Work out the finished part from the listing and answer in its coordinate system (mm). Round coordinates to 2 decimals unless told otherwise and drop trailing zeros. Write each loop counter-clockwise with the first axis right and the second up, starting at its lowest first coordinate (ties: lowest second). Pieces come first, ordered by that corner, then holes.
1. Straight lines are drawn through the part: probe 1 along Y at (x, z) = (99.9, 0); probe 2 along X at (y, z) = (11.75, 0); probe 3 along Z at (x, y) = (28.5, 15). For each, find the intervals that lie inside material, in ascending order.
2. Find section B-B (z = 70). Write down the section's boundary in (x, y).
3. Determine the mould class of faces 1 (the face through (-22.025, 12.522, 99.184)), 2 (the face through (-21.199, 12.878, 95.465)), 3 (the face through (-53, 0, -83)) for opening direction X: pulls with the +X half, pulls with the -X half, needs draft (parallel to the pull), parting line crosses it, or undercut.
4. Find section A-A (x = -28.5). Write down the section's boundary in (y, z).
5. Flat-ended cylindrical pins translate along their axes: pin 1 Ø8 at (x, y) = (-51, 14.5) entering from -Z; pin 2 Ø4 at (y, z) = (19, -23) entering from +X; pin 3 Ø1.6 at (y, z) = (6.35, 0) entering from -X; pin 4 Ø1 at (x, y) = (6, 4) entering from -Z. Find the tip coordinate at first contact, or state that the pin passes through.
6. Find section C-C (y = 12.5). Write down the section's boundary in (x, z), and give its area (3 significant figures).
```python
from build123d import *

# Parameters (mm, degrees)
SKETCH1_R           = 101.6
SKETCH1_R_2         = 82.55
BOSS_EXTRUDE1_DEPTH = 25.4
SKETCH2_R           = 97.79
SKETCH2_R_2         = 63.5
CUT_EXTRUDE1_DEPTH  = 50.8
SKETCH3_R           = 0.9
CUT_EXTRUDE2_DEPTH  = 254
CIRPATTERN1_COUNT   = 12


with BuildPart() as part:
    # Sketch1 → Boss-Extrude1 (new body)
    with BuildSketch(Plane(origin=(0, 0, 0), x_dir=(1, 0, 0), z_dir=(0, 1, 0))):
        Circle(SKETCH1_R)
        Circle(SKETCH1_R_2, mode=Mode.SUBTRACT)
    extrude(amount=BOSS_EXTRUDE1_DEPTH)

    # Sketch2 → Cut-Extrude1 (cut)
    with BuildSketch(Plane(origin=(0, 25.4, 0), x_dir=(1, 0, 0), z_dir=(0, 1, 0))):
        Circle(SKETCH2_R)
        Circle(SKETCH2_R_2, mode=Mode.SUBTRACT)
    extrude(amount=-CUT_EXTRUDE1_DEPTH, mode=Mode.SUBTRACT)

    # Sketch3 → Cut-Extrude2 (cut)
    with BuildSketch(Plane.XY):
        with Locations((0, 6.35)):
            Circle(SKETCH3_R)
    cut_extrude2 = extrude(amount=-CUT_EXTRUDE2_DEPTH, mode=Mode.SUBTRACT)

    # CirPattern1: Cut-Extrude2 ×12 about axis
    cirpattern1_axis = Axis((0, 25.4, 0), (0, 1, 0))
    for i in range(1, CIRPATTERN1_COUNT):
        add(cut_extrude2.rotate(cirpattern1_axis, i * 360 / CIRPATTERN1_COUNT), mode=Mode.SUBTRACT)


solid = part.part
```
Worked answers:
1. probe 1: y = 0 to 5.45, 7.25 to 25.4
1. probe 2: x = -101.6 to -97.79, 97.79 to 101.6
1. probe 3: z = -97.52 to -93.54, 93.54 to 97.52
2. outline: (-73.64, 0) - (-68.29, 0) - (-68.29, 25.4) - (-73.64, 25.4) - close; (68.29, 0) - (73.64, 0) - (73.64, 25.4) - (68.29, 25.4) - close
3. face 1: parting line crosses it
3. face 2: undercut
3. face 3: needs draft
4. outline: (0, -97.52) - (25.4, -97.52) - (25.4, -93.54) - (0, -93.54) - close; (0, 93.54) - (25.4, 93.54) - (25.4, 97.52) - (0, 97.52) - close
5. pin 1: stops at z = -90.08
5. pin 2: stops at x = 99.41
5. pin 3: passes through
5. pin 4: stops at z = -101.45
6. outline: circle Ø203.2 at (0, 0); hole circle Ø195.58 at (0, 0)
6. area: 2,390 mm2
